Autodesk Fusion 360 part; units mm, degrees
sketch "Sketch1" plane through (0, 0, 0) normal (0, 1, 0) x (1, 0, 0)
  line L0 (5, 0) -> (7, 0)
  line L1 (7, 0) -> (7, -3)
  line L2 (6.5, -3) -> (6.5, -7)
  line L3 (5.5, -17) -> (5.5, -8)
  line L4 (6.5, -18) -> (6.5, -22)
  arc A0 (3.5, -25) -> (6.5, -22) centre (3.5, -22) ccw
  line L5 (0.5, -18) -> (0.5, -18)
  line L6 (6.5, -18) -> (6.5, -18)
  line L7 (6.5, -7) -> (6.5, -7)
  line L8 (0.5, -7) -> (0.5, -7)
  arc A1 (5.5, -17) -> (6.5, -18) centre (6.5, -17) ccw
  arc A2 (6.5, -7) -> (5.5, -8) centre (6.5, -8) ccw
  line L9 (7, -3) -> (6.5, -3)
  line L10 (0.5, -3) -> (0, -3)
  line L11 (3.5, 0) -> (3.5, -25) construction
  line L12 (3.5, -25) -> (3.5, -1.5)
  arc A3 (3.5, -1.5) -> (5, 0) centre (3.5, 0) ccw
  point P0 (5.5, -7)
  point P1 (1.5, -7)
  point P2 (5.5, -18)
  dimension "d10" = 7
  dimension "d11" = 3
  dimension "d12" = 6
  dimension "d13" = 4
  dimension "d14" = 4
  dimension "d15" = 11
  dimension "d16" = 6
  dimension "d17" = 6
  dimension "d18" = 4
  dimension "d20" = 1
  dimension "d22" = 1
  dimension "d25" = 3
revolve "Revolve1" add sketch "Sketch1" angle 360 about axis through (3.5, 0, 25) along (0, 0, -1)
equation "lifter_tier_one_height = 3 mm"
equation "lifter_tier_one_diameter = 7 mm"
equation "lifter_tier_two_height = 4 mm"
equation "lifter_tier_two_diameter = 6 mm"
equation "lifter_tier_three_height = 11 mm"
equation "lifter_tier_three_diameter = 4 mm"
equation "lifter_tier_three_radius = 1 mm"
equation "lifter_tier_four_diameter = 6 mm"
equation "lifter_tier_four_total_height = 7 mm"
equation "d10 = lifter_tier_one_diameter"
equation "d11 = lifter_tier_one_height"
equation "d12 = lifter_tier_two_diameter"
equation "d13 = lifter_tier_two_height"
equation "d14 = lifter_tier_three_diameter"
equation "d15 = lifter_tier_three_height"
equation "d16 = lifter_tier_four_diameter"
equation "d17 = lifter_tier_four_diameter"
equation "d18 = lifter_tier_four_total_height - ( lifter_tier_four_diameter / 2 )"
equation "d20 = lifter_tier_three_radius"
equation "d22 = lifter_tier_three_radius"
equation "hemispherical_cut_diameter = 3 mm"
equation "d25 = hemispherical_cut_diameter"
For this review, take the finished solid that the model builds, in its own axes (mm). Round coordinates to 2 decimals unless told otherwise and drop trailing zeros. Loops run counter-clockwise (first coordinate to the right, second up) from the corner with the lowest first, then second, coordinate; pieces in that order, holes last. Notation, with made-up numbers: (-22.5, 44.5) - (7.5, 44.5) arc R15 ccw to (7.5, 49.5) - close; hole circle Ø3 at (41.5, 44.25). An arc over 180 degrees is marked (long way). Put each result on its own line as item: value. Start each with the question number.
1. Consider section D-D on z = 17.25. State the section outline as (x, y) points.
2. Mouldability with a two-part tool opening along Z and no side actions: class faces 1 (the cylindrical face through (6.733, -1.341, 1.521)), 2 (the flat face through (3, 2, 0)), 3 (the cylindrical face through (1.9, 1.2, 12.4)) as +Z half, -Z half, draft (parallel to the pull), parting line (faces both ways), or undercut.
3. Consider section C-C on z = 10.5. State the section outline as (x, y) points, plus the area to 3 significant figures.
4. For probe 1 along Y at (x, z) = (2.5, 18.25); probe 2 along Y at (x, z) = (1.75, 7.75); probe 3 along X at (y, z) = (-1, 22), list the stretches that pass through material, from the lowest coordinate up. Write a range as [from, to].
5. Consider section A-A on x = 3.5. State the section outline as (y, z) points.
6. Consider section B-B on y = 0. State the section outline as (x, z) points.
7. Insertion check: P1, Ø2, axis at y = -2.5, z = 20, coming from the +X side; P2, Ø2, axis at y = 0.5, z = 16.5, coming from the -X side; P3, Ø1.5, axis at y = -1, z = 3, coming from the -X side. Each pin has a flat end and moves straight along its axis. Give the tip position at first contact, or say it passes through.
Result sheet:
1. outline: circle Ø4.06 at (3.5, 0)
2. face 1: draft
2. face 2: -Z half
2. face 3: undercut
3. outline: circle Ø4 at (3.5, 0)
3. area: 12.6 mm^2
4. probe 1: [-2.83, 2.83]
4. probe 2: [-1.03, 1.03]
4. probe 3: [0.67, 6.33]
5. outline: (-3.5, 0) - (-1.5, 0) arc R1.5 cw to (1.5, 0) - (3.5, 0) - (3.5, 3) - (3, 3) - (3, 7) arc R1 cw to (2, 8) - (2, 17) arc R1 cw to (3, 18) - (3, 22) arc R3 ccw to (-3, 22) - (-3, 18) arc R1 cw to (-2, 17) - (-2, 8) arc R1 cw to (-3, 7) - (-3, 3) - (-3.5, 3) - close
6. outline: (0, 0) - (2, 0) arc R1.5 cw to (5, 0) - (7, 0) - (7, 3) - (6.5, 3) - (6.5, 7) arc R1 cw to (5.5, 8) - (5.5, 17) arc R1 cw to (6.5, 18) - (6.5, 22) arc R3 ccw to (0.5, 22) - (0.5, 18) arc R1 cw to (1.5, 17) - (1.5, 8) arc R1 cw to (0.5, 7) - (0.5, 3) - (0, 3) - close
7. P1: x = 6.1
7. P2: x = 1.4
7. P3: x = 0.01
